The listing builds one solid part. Answer for the finished solid, in the listing's coordinates (mm). A direction names the side the tool comes from. Round coordinates to 2 decimals unless told otherwise and drop trailing zeros. Order: outer loops, then holes, each group sorted by start corner. A loop starts at its lowest first (then second) coordinate and runs counter-clockwise, first axis right, second up. Notation, with made-up numbers: (60.25, 84.5) -> (66.25, 84.5) arc R5 cw to (66.25, 92.5) -> close; hole circle Ø2 at (33.5, 41.25). An arc over 180 degrees is marked (long way). Answer in a Markdown table with one row per item. Add a question column.
```python
from build123d import *

# Parameters (mm, degrees)
F0_W     = 150.5499258637
F0_H     = 101.7426103354
F1_DEPTH = 50.8
F3_DEPTH = 50.8
F5_DEPTH = 50.8
F7_DEPTH = 25.4


with BuildPart() as f1:
    # F0 (on Front) → F1 (new body)
    with BuildSketch(Plane.XZ):
        with Locations((-0.8498765528, 5.2206814289)):
            Rectangle(F0_W, F0_H)
    extrude(amount=F1_DEPTH)

    # F2 (on face) → F3 (cut)
    with BuildSketch(Plane(origin=(-76.1248394847, 0, 0), x_dir=(0, -1, 0), z_dir=(-1, 0, 0))):
        Polygon((0, 56.0919865966), (50.8, -19.1829744726), (50.8, 56.0919865966), align=None)
    extrude(amount=-F3_DEPTH, mode=Mode.SUBTRACT)

    # F4 (on face) → F5 (cut)
    with BuildSketch(Plane.YZ.offset(74.4250863791)):
        Polygon((-50.8, 56.0919865966), (-50.8, -19.4257982075), (0, 56.0919865966), align=None)
    extrude(amount=-F5_DEPTH, mode=Mode.SUBTRACT)

    # F6 (on face) → F7 (join)
    with BuildSketch(Plane(origin=(0, 0, 0), x_dir=(-1, 0, 0), z_dir=(0, 1, 0))):
        Polygon((-23.6250863791, 56.0919865966), (-74.4250863791, 56.0919865966), (-74.4250863791, -45.6506237388), (76.1248394847, -45.6506237388), (76.1248394847, 56.0919865966), (25.3248394847, 56.0919865966), align=None)
    extrude(amount=F7_DEPTH)


solid = f1.part
```
1. Straight lines are drawn through the part: line 1 along Y through (x, z) = (-67, -11.5); line 2 along Z through (x, y) = (57, -11.5); line 3 along Z through (x, y) = (-50.5, -4). For each, find the intervals that lie inside material, in ascending order.
2. The part is cut by section C-C (x = 49.5). Give the vertices of the cut face in (y, z).
3. The part is cut by section B-B (z = 7.5). Give the vertices of the cut face in (x, y).
4. For faces 1 (the flat face through (23.625, -31, 27)), 2 (the flat face through (-2, -50.8, -5)), 3 (the flat face through (-51.08, -25.044, 18.981)), determine the directions among +Z, -Z, +X, -X, +Y, -Y from which every point of the face is accessible in a straight line to the end or side of a thin tool.
5. The part is cut by section D-D (x = -56.5). Give the vertices of the cut face in (y, z).
6. Each of these flat-tipped pins is pushed along its axis until it touches: pin 1 (10 mm diameter, centred on y = -37.5, z = 10.5, fed in from +X); pin 2 (6 mm diameter, centred on y = -29.5, z = 24, fed in from -X). Where does it stop, or does it pass through?
7. The part is cut by section A-A (y = -22). Give the vertices of the cut face in (x, z).
Report:
| question | item | result |
|---|---|---|
| 1 | line 1 | y = -45.62 to 25.4 |
| 1 | line 2 | z = -45.65 to 39 |
| 1 | line 3 | z = -45.65 to 50.16 |
| 2 | outline | (-50.8, -45.65) -> (25.4, -45.65) -> (25.4, 56.09) -> (0, 56.09) -> (-50.8, -19.43) -> close |
| 3 | outline | (-76.12, -32.79) -> (-25.32, -32.79) -> (-25.32, -50.8) -> (23.63, -50.8) -> (23.63, -32.69) -> (74.43, -32.69) -> (74.43, 25.4) -> (-76.12, 25.4) -> close |
| 4 | face 1 | +Z, +X, -Y |
| 4 | face 2 | +Z, -Z, +X, -X, -Y |
| 4 | face 3 | +Z, -X, -Y |
| 5 | outline | (-50.8, -45.65) -> (25.4, -45.65) -> (25.4, 56.09) -> (0, 56.09) -> (-50.8, -19.18) -> close |
| 6 | pin 1 | stops at x = 23.63 |
| 6 | pin 2 | stops at x = -25.32 |
| 7 | outline | (-76.12, -45.65) -> (74.43, -45.65) -> (74.43, 23.39) -> (23.63, 23.39) -> (23.63, 56.09) -> (-25.32, 56.09) -> (-25.32, 23.49) -> (-76.12, 23.49) -> close |
